Read the model definition and answer for the solid it produces. Units are mm, in the model's axes. A direction names the side the tool comes from. Coordinates: 2 decimals unless noted, no trailing zeros. Loops run counter-clockwise (first coordinate to the right, second up) from the corner with the lowest first, then second, coordinate; pieces in that order, holes last. Notation, with made-up numbers: (41, 64) - (82, 64) arc R19 cw to (82, 76) - close; hole circle Ø2 at (74.5, -17.75). An arc over 180 degrees is marked (long way). One line per item, written item: value. Start each with the question number.
from build123d import *

# Parameters (mm, degrees)
BOSS_EXTRUDE1_DEPTH = 8
SKETCH2_R           = 1.190625
CUT_EXTRUDE1_DEPTH  = 15.990663761
FILLET1_R           = 1
FILLET2_R           = 1
SKETCH3_W           = 4.5
SKETCH3_H           = 0.2
CUT_EXTRUDE2_DEPTH  = 10


with BuildPart() as part:
    # Sketch1 → Boss-Extrude1 (new body)
    with BuildSketch(Plane.XY):
        Polygon((0, 0), (8, 0), (11.5, -3.5), (17.5, -3.5), (17.5, -3.7), (11.417157288, -3.7), (7.917157288, -0.2), (0.082842712, -0.2), (-3.417157288, -3.7), (-9.5, -3.7), (-9.5, -3.5), (-3.5, -3.5), align=None)
    extrude(amount=BOSS_EXTRUDE1_DEPTH)

    # Sketch2 → Cut-Extrude1 (cut, through all)
    with BuildSketch(Plane(origin=(0, 0, 0), x_dir=(0, 0, 1), z_dir=(-0.707106781, 0.707106781, 0))):
        with Locations((2.25, -2.5)):
            Circle(SKETCH2_R)
        with Locations((5.75, -2.5)):
            Circle(SKETCH2_R)
    extrude(amount=-CUT_EXTRUDE1_DEPTH, mode=Mode.SUBTRACT)

    # Fillet1
    fillet1_edges = [part.edges().sort_by_distance(p)[0] for p in [
        (0, 0, 4),
        (8, 0, 4),
        (11.5, -3.5, 4),
        (11.417157288, -3.7, 4),
        (7.917157288, -0.2, 4),
        (0.082842712, -0.2, 4),
        (-3.417157288, -3.7, 4),
        (-3.5, -3.5, 4),
    ]]
    fillet(fillet1_edges, radius=FILLET1_R)

    # Fillet2
    fillet2_edges = [part.edges().sort_by_distance(p)[0] for p in [
        (-9.5, -3.6, 8),
        (17.5, -3.6, 0),
        (-9.5, -3.6, 0),
        (17.5, -3.6, 8),
    ]]
    fillet(fillet2_edges, radius=FILLET2_R)

    # Sketch3 → Cut-Extrude2 (cut)
    with BuildSketch(Plane(origin=(0, -3.5, 0), x_dir=(1, 0, 0), z_dir=(0, 1, 0))):
        with Locations((-7.25, -4)):
            Rectangle(SKETCH3_W, SKETCH3_H)
    cut_extrude2 = extrude(amount=-CUT_EXTRUDE2_DEPTH, mode=Mode.SUBTRACT)

    # Mirror1: Cut-Extrude2 across plane
    add(cut_extrude2.mirror(Plane(origin=(4, 0, 0), x_dir=(0, 0, 1), z_dir=(1, 0, 0))), mode=Mode.SUBTRACT)


solid = part.part
1) Flat-ended cylindrical pins translate along their axes: P1, Ø2, axis at x = -1.5, z = 5, coming from the -Y side; P2, Ø4.5, axis at x = 15.5, z = 4, coming from the +Y side. Find the tip coordinate at first contact, or state that the pin passes through.
2) Straight lines are drawn through the part: L1, parallel to Y at x = 12, z = 6.25; L2, parallel to Y at x = 1.5, z = 5.75; L3, parallel to X at y = -0.5, z = 5. For each, find the intervals that lie inside material, in ascending order.
3) For faces 4 (the flat face through (15, -3.7, 3)), 5 (the flat face through (15, -3.5, 5)), 6 (the flat face through (-1.647, -1.93, 3.944)), determine the directions among +Z, -Z, +X, -X, +Y, -Y from which every point of the face is accessible in a straight line to the end or side of a thin tool.
4) Section C-C, the plane z = 0.5 is taken. Determine the outline of the cut face in (x, y).
5) Determine the mould class of faces 1 (the flat face through (-2, -2, 4)), 2 (the flat face through (-7, -3.5, 3)), 3 (the flat face through (4, -0.2, 4)) for opening direction X: released by +X, released by -X, zero draft, split by the parting line, or undercut.
6) Section B-B, the plane z = 5 is taken. Determine the outline of the cut face in (x, y).
7) Section D-D, the plane y = -2.35 is taken. State how many separate pieces and enclosed holes the cut face has, and give its area (3 significant figures).
8) Section A-A, the plane x = -7.25 is taken. Determine the outline of the cut face in (y, z), and give its area (3 significant figures).
Answer below:
1. P1: y = -2.78
1. P2: y = -3.5
2. L1: -3.7 to -3.5
2. L2: -0.2 to 0
2. L3: -0.5 to -0.22, 8.22 to 8.5
3. face 4: +Z, -Z, +X, -X, -Y
3. face 5: +Z, -Z, +X, +Y
3. face 6: +Z, -Z, -Y
4. outline: (-9.37, -3.7) - (-3.83, -3.7) arc R1 ccw to (-3.12, -3.41) - (-0.21, -0.49) arc R1 cw to (0.5, -0.2) - (7.5, -0.2) arc R1 cw to (8.21, -0.49) - (11.12, -3.41) arc R1 ccw to (11.83, -3.7) - (17.37, -3.7) - (17.37, -3.5) - (11.91, -3.5) arc R1 cw to (11.21, -3.21) - (8.29, -0.29) arc R1 ccw to (7.59, 0) - (0.41, 0) arc R1 ccw to (-0.29, -0.29) - (-3.21, -3.21) arc R1 cw to (-3.91, -3.5) - (-9.37, -3.5) - close
5. face 1: released by -X
5. face 2: zero draft
5. face 3: undercut
6. outline: (-9.5, -3.7) - (-3.83, -3.7) arc R1 ccw to (-3.12, -3.41) - (-2.28, -2.56) - (-2.42, -2.42) - (-3.21, -3.21) arc R1 cw to (-3.91, -3.5) - (-9.5, -3.5) - close; (-1.11, -1.11) - (-0.97, -1.26) - (-0.21, -0.49) arc R1 cw to (0.5, -0.2) - (7.5, -0.2) arc R1 cw to (8.21, -0.49) - (11.12, -3.41) arc R1 ccw to (11.83, -3.7) - (17.5, -3.7) - (17.5, -3.5) - (11.91, -3.5) arc R1 cw to (11.21, -3.21) - (8.29, -0.29) arc R1 ccw to (7.59, 0) - (0.41, 0) arc R1 ccw to (-0.29, -0.29) - close
7. separate pieces: 4
7. enclosed holes: 0
7. area: 3.46 mm2
8. outline: (-3.7, 0) - (-3.5, 0) - (-3.5, 3.9) - (-3.7, 3.9) - close; (-3.7, 4.1) - (-3.5, 4.1) - (-3.5, 8) - (-3.7, 8) - close
8. area: 1.56 mm2
